Here's how the part is built. I have some questions about the finished solid (model axes, mm). Face numbers are marked on the shaded views. A direction names the side the tool comes from. Give positions to 0.01 mm unless a question says otherwise; leave off trailing zeros. Loops run counter-clockwise (first coordinate to the right, second up) from the corner with the lowest first, then second, coordinate; pieces in that order, holes last. Notation, with made-up numbers: (-12.75, 67) - (28.25, 67) arc R15 ccw to (28.25, 87) - close; hole circle Ø5 at (20.5, 1). An arc over 180 degrees is marked (long way). Use a Markdown table: item, result.
from build123d import *

# Parameters (mm, degrees)
F2_R     = 12.7
F3_DEPTH = 1.27
F4_R     = 12.7
F5_DEPTH = 1.27
F7_R     = 3.175
F8_DEPTH = 12.7


with BuildPart() as f1:
    # F0 (on Front) → F1 (revolve)
    with BuildSketch(Plane.XZ):
        Polygon((0, 3.437184), (0, 16.137184), (-12.7, 16.137184), (-6.35, 9.787184), (-12.7, 3.437184), (-6.35, 3.437184), align=None)
    revolve(axis=Axis((0, 0, 9.787184), (0, 0, -1)))

    # F2 (on face) → F3 (join)
    with BuildSketch(Plane.XY.offset(16.137184)):
        Circle(F2_R)
    extrude(amount=F3_DEPTH)

    # F4 (on face) → F5 (join)
    with BuildSketch(Plane(origin=(0, 0, 3.437184), x_dir=(1, 0, 0), z_dir=(0, 0, -1))):
        Circle(F4_R)
    extrude(amount=F5_DEPTH)

    # F7 (on face) → F8 (cut)
    with BuildSketch(Plane.XY.offset(17.407184)):
        Circle(F7_R)
    extrude(amount=-F8_DEPTH, mode=Mode.SUBTRACT)


solid = f1.part
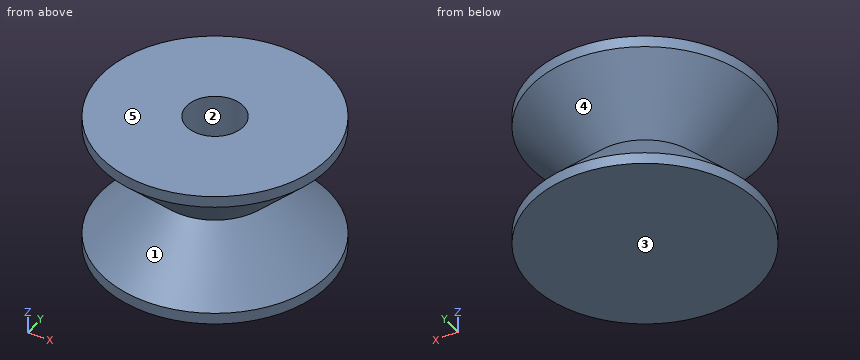
(1) Suppose I cut it at A-A on x = 0. Write out the boundary of the cut face in (y, z) (3 decimals).
A:
| item | result |
|---|---|
| outline | (-12.7, 2.167) - (12.7, 2.167) - (12.7, 3.437) - (6.35, 9.787) - (12.7, 16.137) - (12.7, 17.407) - (3.175, 17.407) - (3.175, 4.707) - (-3.175, 4.707) - (-3.175, 17.407) - (-12.7, 17.407) - (-12.7, 16.137) - (-6.35, 9.787) - (-12.7, 3.437) - close |
(2) Suppose I cut it at D-D on z = 15.75. Write out the boundary of the cut face in (x, y) (3 decimals).
A:
| item | result |
|---|---|
| outline | circle Ø24.626 at (0, 0); hole circle Ø6.35 at (0, 0) |
(3) On a 3-axis mill with a long thin cutter (end or side, diameter ignored), from which of +Z, -Z, +X, -X, +Y, -Y can I reach the whole of each face in a straight line? I mean the marked faces 4 and 5. Say none if no direction works.
A:
| item | result |
|---|---|
| face 4 | none |
| face 5 | +Z, +X, -X, +Y, -Y |
(4) If I drill on line 1 (Z direction, x = -1.25, y = 0.5); line 2 (Z direction, x = 7.75, y = -9.75); line 3 (Z direction, x = -2.5, y = 8.75), over which ranges is the centre line in solid material (lowest first)?
A:
| item | result |
|---|---|
| line 1 | 2.17 to 4.71 |
| line 2 | 2.17 to 3.68, 15.89 to 17.41 |
| line 3 | 2.17 to 7.04, 12.54 to 17.41 |
(5) We'd pull the mould along X, two halves only. Please class the marked faces 1, 2 and 3: pulls with the +X half, pulls with the -X half, needs draft (parallel to the pull), parting line crosses it, or undercut.
A:
| item | result |
|---|---|
| face 1 | parting line crosses it |
| face 2 | undercut |
| face 3 | needs draft |
(6) Suppose I cut it at C-C on z = 9.25. Write out the boundary of the cut face in (x, y) (3 decimals), plus the area to 3 significant figures.
A:
| item | result |
|---|---|
| outline | circle Ø13.774 at (0, 0); hole circle Ø6.35 at (0, 0) |
| area | 117 mm2 |
(7) Will these pins go through, and if not, where does the flat tip stop? pin 1 (4 mm diameter, centred on y = -2, z = 15, fed in from -X); pin 2 (7 mm diameter, centred on x = -0.5, y = 1.5, fed in from +Z); pin 3 (3 mm diameter, centred on x = -1, z = 7, fed in from +Y); pin 4 (4 mm diameter, centred on x = 4.5, z = 15.5, fed in from +Y).
A:
| item | result |
|---|---|
| pin 1 | x = -12.7 |
| pin 2 | z = 17.41 |
| pin 3 | y = 10.6 |
| pin 4 | y = 12.43 |
